Part model, mm, in its own coordinate system. Face numbers are marked on the shaded views. A direction names the side the tool comes from. Coordinates: 2 decimals unless noted, no trailing zeros. Loops run counter-clockwise (first coordinate to the right, second up) from the corner with the lowest first, then second, coordinate; pieces in that order, holes last. Notation, with made-up numbers: (21, -37.75) -> (52, -37.75) arc R15 ccw to (52, -15.75) -> close; hole circle Ø9 at (-27.75, -12.5). An arc over 180 degrees is marked (long way). Use one line per item in the form item = value. Start each with the question number.
(1) Band-saw the part on A-A on y = 38. Give the cut face in (x, z).
(2) Band-saw the part on B-B on y = 14. Give the cut face in (x, z), then the cut area to 3 significant figures.
(3) 3-axis set-ups, long thin cutter, end or side, ignore diameter. For the marked faces 1, 2 and 3: which of +Z, -Z, +X, -X, +Y, -Y reach the whole face in a straight line?
(4) Pin check, flat tips, straight feed: P1, Ø3, axis at x = 0, z = -9.5, coming from the -Y side; P2, Ø3, axis at x = 9, y = 24.5, coming from the +Z side; P3, Ø1.5, axis at x = -7, y = 27.5, coming from the +Z side. Stop position of each tip, or through.
(5) Drill centre lines: L1, parallel to Y at x = 8.5, z = 0.75; L2, parallel to Z at x = 0, y = 27.25; L3, parallel to Y at x = 5.75, z = 2.25. Where is each one in solid material? Low to high. Write a range as [from, to].
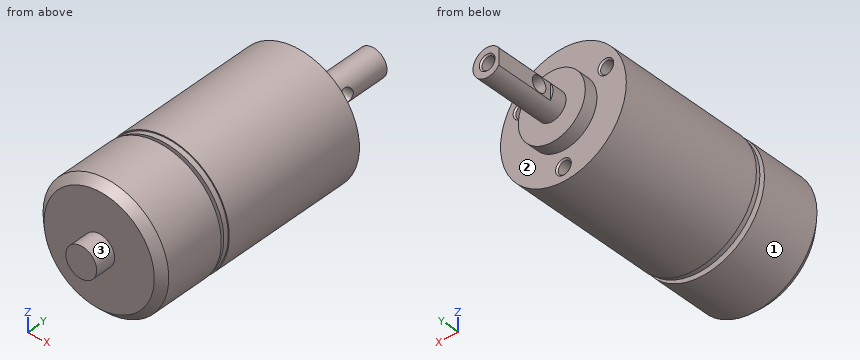
```python
from build123d import *

# Parameters (mm, degrees)
SKETCH_2_R                   = 2.75
EXTRUDE_1_DEPTH              = 14.4
CUT_EXTRUDE_1_DEPTH          = 51.066755437
CUT_EXTRUDE_1_DEPTH_BACK     = 51.066755437
SKETCH_3_W                   = 1.5
SKETCH_3_H                   = 12
CUT_EXTRUDE_2_REACH          = 52.662
CUT_EXTRUDE_2_END_RADIUS     = 2.75
SKETCH_4_R                   = 1.5
HOLE_WIZARD_M3_1_D           = 2.5
HOLE_WIZARD_M3_1_DEPTH       = 5.5
HOLE_WIZARD_M3_1_CSINK_D     = 3.05
HOLE_WIZARD_M3_1_CSINK_ANGLE = 90
HOLE_WIZARD_M3_1_TIP         = 0.751075774
HOLE_WIZARD_M3_2_D           = 2.5
HOLE_WIZARD_M3_2_DEPTH       = 4
HOLE_WIZARD_M3_2_CSINK_D     = 3.05
HOLE_WIZARD_M3_2_CSINK_ANGLE = 90
HOLE_WIZARD_M3_2_TIP         = 0.751075774
CHAMFER_1_SIZE               = 1.5
SKETCH_9_R                   = 3
EXTRUDE_2_DEPTH              = 4


with BuildPart() as part:
    # 草图1 → 旋转1 (revolve)
    with BuildSketch(Plane.XY, mode=Mode.PRIVATE) as revolve_1_sk:
        Polygon((3, 0), (12, 0), (12, 1), (12.2, 1), (12.2, 30), (6.5, 30), (6.5, 32.6), (0, 32.6), (0, -14), (12.2, -14), (12.2, -0.8), (3, -0.8), align=None)
    revolve(revolve_1_sk.sketch.rotate(Axis((0, 32.6, 0), (0, -1, 0)), 180), axis=Axis((0, 32.6, 0), (0, -1, 0)))

    # 草图2 → 凸台-拉伸1 (add)
    with BuildSketch(Plane(origin=(0, 32.6, 0), x_dir=(1, 0, 0), z_dir=(0, 1, 0))):
        Circle(SKETCH_2_R)
    extrude(amount=EXTRUDE_1_DEPTH)

    # 草图3 → 切除-拉伸1 (cut, two sides: drawn at the far end of the back side and taken through both)
    with BuildSketch(Plane.XY.offset(-CUT_EXTRUDE_1_DEPTH_BACK)):
        with Locations((-3, 41.5)):
            Rectangle(SKETCH_3_W, SKETCH_3_H)
    extrude(amount=CUT_EXTRUDE_1_DEPTH + CUT_EXTRUDE_1_DEPTH_BACK, mode=Mode.SUBTRACT)

    # 切除-拉伸2: up to this cylinder (the profile starts inside it)
    cut_extrude_2_end = Plane(origin=(0, 38, 0), z_dir=(0, -1, 0)) * Cylinder(CUT_EXTRUDE_2_END_RADIUS, 111.824, mode=Mode.PRIVATE)
    # 草图4 → 切除-拉伸2 (cut, up to the surface)
    with BuildSketch(Plane.ZY.offset(2.25), mode=Mode.PRIVATE) as cut_extrude_2_sk1:
        with Locations(Location((0, 38, 0), (0, 0, 270))):
            Circle(SKETCH_4_R)
    cut_extrude_2_tool1 = extrude(cut_extrude_2_sk1.sketch, amount=-CUT_EXTRUDE_2_REACH, mode=Mode.PRIVATE) & cut_extrude_2_end
    add(cut_extrude_2_tool1.solids().sort_by_distance((-2.25, 38, 0))[0], mode=Mode.SUBTRACT)

    # M3 螺纹孔1
    with Locations(Plane(origin=(0, 47, 0), x_dir=(1, 0, 0), z_dir=(0, 1, 0))):
        with Locations((0, 0)):
            CounterSinkHole(HOLE_WIZARD_M3_1_D / 2, HOLE_WIZARD_M3_1_CSINK_D / 2, depth=HOLE_WIZARD_M3_1_DEPTH, counter_sink_angle=HOLE_WIZARD_M3_1_CSINK_ANGLE)
            with Locations((0, 0, -(HOLE_WIZARD_M3_1_DEPTH + HOLE_WIZARD_M3_1_TIP / 2))):  # 118° drill point
                Cone(0, HOLE_WIZARD_M3_1_D / 2, HOLE_WIZARD_M3_1_TIP, mode=Mode.SUBTRACT)

    # M3 螺纹孔2
    with Locations(Plane(origin=(8.227241336, 30, 4.75), x_dir=(1, 0, 0), z_dir=(0, 1, 0))):
        with Locations((0, 0), (-16.454482672, 0), (-8.227241336, 14.25)):
            CounterSinkHole(HOLE_WIZARD_M3_2_D / 2, HOLE_WIZARD_M3_2_CSINK_D / 2, depth=HOLE_WIZARD_M3_2_DEPTH, counter_sink_angle=HOLE_WIZARD_M3_2_CSINK_ANGLE)
            with Locations((0, 0, -(HOLE_WIZARD_M3_2_DEPTH + HOLE_WIZARD_M3_2_TIP / 2))):  # 118° drill point
                Cone(0, HOLE_WIZARD_M3_2_D / 2, HOLE_WIZARD_M3_2_TIP, mode=Mode.SUBTRACT)

    # 倒角1
    chamfer_1_edges = [part.edges().sort_by_distance(p)[0] for p in [
        (12.2, -14, 0),
    ]]
    chamfer(chamfer_1_edges, length=CHAMFER_1_SIZE)

    # 草图9 → 凸台-拉伸2 (add)
    with BuildSketch(Plane.XZ.offset(14)):
        with Locations(Location((0, 0, 0), (0, 0, 180))):
            Circle(SKETCH_9_R)
    extrude(amount=EXTRUDE_2_DEPTH)


solid = part.part
```
A:
q1.outline = (-2.25, -1.58) arc R2.75 ccw to (2.3, -1.5) -> (-2.25, -1.5) -> close; (-2.25, 1.5) -> (2.3, 1.5) arc R2.75 ccw to (-2.25, 1.58) -> close
q2.outline = circle Ø24.4 at (0, 0)
q2.area = 468 mm²
q3.face_1 = +Y, -Y
q3.face_2 = +Y
q3.face_3 = -Y
q4.P1 = -14
q4.P2 = 9.62
q4.P3 = 10.48
q5.L1 = [-14, -0.8], [0, 30]
q5.L2 = [-12.2, -10.75], [-8.25, 12.2]
q5.L3 = [-14, -0.8], [0, 32.6]
